Autodesk Inventor part; units mm, degrees
ref_plane "YZ Plane" through (0, 0, 0) normal (1, 0, 0) x (0, 1, 0)
ref_plane "XZ Plane" through (0, 0, 0) normal (0, 1, 0) x (-1, 0, 0)
ref_plane "XY Plane" through (0, 0, 0) normal (0, 0, 1) x (1, 0, 0)
sketch "Sketch1" plane through (0, 0, 0) normal (0, 0, 1) x (1, 0, 0)
  circle A0 centre (0, 0) radius 12.5
  dimension "d0" = 25
extrude "Extrusion1" add sketch "Sketch1" along normal blind 1.5
sketch "Sketch2" plane through (0, 0, 0) normal (0, 0, -1) x (-1, 0, 0)
  circle A0 centre (0, 0) radius 12.5
  circle A1 centre (0, 0) radius 11
  dimension "d3" = 22
extrude "Extrusion2" add sketch "Sketch2" along normal blind 6.5 contours A1
sketch "Sketch3" plane through (0, 0, -6.5) normal (0, 0, -1) x (-1, 0, 0)
  circle A0 centre (0, 0) radius 11
  circle A1 centre (0, 0) radius 12.5
  dimension "d6" = 25
extrude "Extrusion3" add sketch "Sketch3" along normal blind 1.5 contours A0 | A1
sketch "Sketch4" plane through (0, 0, -8) normal (0, 0, -1) x (-1, 0, 0)
  circle A0 centre (0, 0) radius 12.5
  circle A1 centre (0, 3.5) radius 4.75
  dimension "d9" = 3.5
  dimension "d10" = 9.5
extrude "Extrusion4" cut sketch "Sketch4" against normal through all contours A1
sketch "Sketch6" plane through (0, 0, 0) normal (0, 1, 0) x (-1, 0, 0)
  line L0 (11, 0) -> (11, -6.5)
  line L1 (-11, 0) -> (-11, -6.5)
  line L2 (-12.5, -6.5) -> (12.5, -6.5)
  point P0 (0, 0)
  point P1 (0, -3.25)
  point P2 (11, -3.25)
  dimension "d18" = 11
  dimension "d19" = 3.25
hole "Hole1" at (0, 0, -3.25) direction (0, -1, 0) diameter 2.459 end through all
chamfer "Chamfer1" distance 0.1 angle 45 2 edges at (12.5, 0, -8) (-12.5, 0, 1.5)
properties part number "28 - Eccentric  Sheav" material "Steel AISI 1020 108 ANLD"
The listing builds one solid part. Answer for the finished solid, in the listing's coordinates (mm). A direction names the side the tool comes from. Give positions to 0.01 mm unless a question says otherwise; leave off trailing zeros. Order: outer loops, then holes, each group sorted by start corner. A loop starts at its lowest first (then second) coordinate and runs counter-clockwise, first axis right, second up. Notation, with made-up numbers: (30, 3.5) -> (58, 3.5) arc R15 cw to (58, 21.5) -> close; hole circle Ø5 at (22.25, 24). An arc over 180 degrees is marked (long way). Put each result on its own line as item: value.
Item 1: Given P1, Ø1.5, axis at y = 9, z = -1.5, coming from the -X side; P2, Ø3, axis at x = 8.5, z = -2, coming from the -Y side; P3, Ø1.5, axis at x = 2.5, y = 5, coming from the +Z side; P4, Ø3, axis at y = -9.5, z = -7, coming from the +X side, each flat-ended and moving along its own axis, determine where each tip first touches the part or whether it passes through.
Established:
P1: stops at x = -7.28
P2: stops at y = -8.49
P3: passes through
P4: stops at x = 9.6
Item 2: A cutting plane is placed at C-C on z = -3.25. Give the vertices of the cut face in (x, y), plus the area to 3 significant figures.
Established:
outline: (-1.23, -10.93) -> (-1.23, -1.09) arc R4.75 cw (long way) to (1.23, -1.09) -> (1.23, -10.93) arc R11 ccw (long way) to start
area: 285 mm^2
Item 3: A cutting plane is placed at A-A on x = 0. Give the vertices of the cut face in (y, z), plus the area to 3 significant figures.
Established:
outline: (-12.5, -7.9) -> (-12.4, -8) -> (-1.25, -8) -> (-1.25, -4.48) -> (-11, -4.48) -> (-11, -6.5) -> (-12.5, -6.5) -> close; (-12.5, 0) -> (-11, 0) -> (-11, -2.02) -> (-1.25, -2.02) -> (-1.25, 1.5) -> (-12.4, 1.5) -> (-12.5, 1.4) -> close; (8.25, -8) -> (12.4, -8) -> (12.5, -7.9) -> (12.5, -6.5) -> (11, -6.5) -> (11, 0) -> (12.5, 0) -> (12.5, 1.4) -> (12.4, 1.5) -> (8.25, 1.5) -> close
area: 104 mm^2
Item 4: For faces 1 (the face through (-2.554, 7.505, -3.317)), 2 (the face through (0.748, -6.113, -4.226)), 3 (the face through (5, -10, 0)), determine the directions among +Z, -Z, +X, -X, +Y, -Y from which every point of the face is accessible in a straight line to the end or side of a thin tool.
Established:
face 1: +Z, -Z
face 2: -Y
face 3: none
Item 5: A cutting plane is placed at B-B on z = -6. Give the vertices of the cut face in (x, y), plus the area to 3 significant figures.
Established:
outline: circle Ø22 at (0, 0); hole circle Ø9.5 at (0, 3.5)
area: 309 mm^2
Item 6: For a pull along Z with two mould halves and no side action, classify faces 4 (the face through (-11.923, -3.755, -7.19)), 5 (the face through (2.38, 10.74, -3.2)), 6 (the face through (0, -3, -8)), 7 (the face through (0, -3, 1.5)) as released by +Z, released by -Z, zero draft, split by the parting line, or undercut.
Established:
face 4: zero draft
face 5: undercut
face 6: released by -Z
face 7: released by +Z
Item 7: Straight lines are drawn through the part: line 1 (Y direction, x = 0, z = -1.75); line 2 (Y direction, x = -0.25, z = 0.75); line 3 (Z direction, x = 0, y = -4). For each, find the intervals that lie inside material, in ascending order.
Established:
line 1: y = -11 to -1.25, 8.25 to 11
line 2: y = -12.5 to -1.24, 8.24 to 12.5
line 3: z = -8 to -4.48, -2.02 to 1.5
